The listing builds one solid part. Answer for the finished solid, in the listing's coordinates (mm). A direction names the side the tool comes from. Give positions to 0.01 mm unless a question says otherwise; leave off trailing zeros. Write each loop counter-clockwise with the first axis right and the second up, starting at its lowest first coordinate (ties: lowest second). Pieces come first, ordered by that corner, then holes. Notation, with made-up numbers: M -37,0 L -31,0 A25 cw -31,28 Z; hole C -9,42.25 d5. An arc over 180 degrees is marked long. Return JSON: item names as keys, results as strings.
from build123d import *

# Parameters (mm, degrees)
EXTRUDE_1_DEPTH = 7


with BuildPart() as part:
    # 草图2 → 凸台-拉伸1 (new body)
    with BuildSketch(Plane(origin=(0, 0, 0), x_dir=(1, 0, 0), z_dir=(0, 1, 0))):
        with BuildLine():
            Line((0, 0), (7, 0))
            ThreePointArc((7, 0), (8.414213562, 0.585786438), (9, 2))
            Line((9, 2), (9, 46.39280404))
            ThreePointArc((9, 46.39280404), (8.811088093, 48.327371287), (8.251489914, 50.188845976))
            ThreePointArc((8.251489914, 50.188845976), (7.689663967, 52.057731217), (7.5, 53.999999998))
            Line((7.5, 53.999999998), (7.5, 67.999999998))
            ThreePointArc((7.5, 67.999999998), (6.914213562, 69.41421356), (5.5, 69.999999998))
            Line((5.5, 69.999999998), (0, 69.999999998))
            Line((0, 69.999999998), (-5.5, 69.999999998))
            ThreePointArc((-5.5, 69.999999998), (-6.914213562, 69.41421356), (-7.5, 67.999999998))
            Line((-7.5, 67.999999998), (-7.5, 53.999999998))
            ThreePointArc((-7.5, 53.999999998), (-7.689663967, 52.057731217), (-8.251489914, 50.188845976))
            ThreePointArc((-8.251489914, 50.188845976), (-8.811088093, 48.327371287), (-9, 46.39280404))
            Line((-9, 46.39280404), (-9, 2))
            ThreePointArc((-9, 2), (-8.414213562, 0.585786438), (-7, 0))
            Line((-7, 0), (0, 0))
        make_face()
    extrude(amount=EXTRUDE_1_DEPTH)


solid = part.part
Item 1: Given pin 1 Ø2 at (y, z) = (2, -58.5) entering from -X, flat-ended and moving along its own axis, determine where the tip first touches the part or whether it passes through.
Geometry results:
{"pin 1": "stops at x = -7.5"}
Item 2: A cutting plane is placed at B-B, the plane z = -63.5. Write down the section's boundary in (x, y).
Geometry results:
{"outline": "M -7.5,0 L 7.5,0 L 7.5,7 L -7.5,7 Z"}
Item 3: A cutting plane is placed at C-C, the plane z = -51.5. Write down the section's boundary in (x, y), plus the area to 3 significant figures.
Geometry results:
{"outline": "M -7.82,0 L 7.82,0 L 7.82,7 L -7.82,7 Z", "area": "109 mm2"}
Item 4: Which of the six approach directions +Z, -Z, +X, -X, +Y, -Y give full straight-line access (tool end or side, diameter ignored) to faces 1 (the flat face through (7.5, 3, -61)), 2 (the flat face through (-7.5, 3, -61)), 3 (the cylindrical face through (-8.43, 3.45, -0.6))?
Geometry results:
{"face 1": "-Z, +X, +Y, -Y", "face 2": "-Z, -X, +Y, -Y", "face 3": "+Z, -X, +Y, -Y"}
Item 5: Find the intervals of material crossed by line 1 (X direction, y = 6.25, z = -64); line 2 (X direction, y = 2.5, z = -46.5), in increasing order.
Geometry results:
{"line 1": "x = -7.5 to 7.5", "line 2": "x = -9 to 9"}
Item 6: A cutting plane is placed at A-A, the plane y = 1.5. Write down the section's boundary in (x, z).
Geometry results:
{"outline": "M -9,-46.39 A10 ccw -8.25,-50.19 A10.04 cw -7.5,-54 L -7.5,-68 A2 ccw -5.5,-70 L 5.5,-70 A2 ccw 7.5,-68 L 7.5,-54 A10.04 cw 8.25,-50.19 A10 ccw 9,-46.39 L 9,-2 A2 ccw 7,0 L -7,0 A2 ccw -9,-2 Z"}
